Autodesk Inventor part; units mm, degrees
ref_plane "YZ Plane" through (0, 0, 0) normal (1, 0, 0) x (0, 1, 0)
ref_plane "XZ Plane" through (0, 0, 0) normal (0, 1, 0) x (-1, 0, 0)
ref_plane "XY Plane" through (0, 0, 0) normal (0, 0, 1) x (1, 0, 0)
sketch "Sketch1" plane through (0, 0, 0) normal (0, 1, 0) x (-1, 0, 0)
  line L0 (0, 0) -> (0, 10)
  line L1 (0, 10) -> (18.8, 10)
  line L2 (18.8, 10) -> (18.8, 5)
  line L3 (18.8, 5) -> (32.9, 5)
  line L4 (32.9, 5) -> (32.9, 0)
  line L5 (32.9, 0) -> (0, 0)
  dimension "d0" = 65.8
  dimension "d1" = 37.6
  dimension "d2" = 5
  dimension "d3" = 5
revolve "Revolution1" add sketch "Sketch1" angle 360 about axis through (0, 0, 0) along (0, 0, 1)
hole "Hole1" at (0, 0, 0) direction (0, 0, 1) diameter 25 end through all
chamfer "Chamfer1" distance 0.5 angle 45 4 edges at (32.9, 0, 0) (18.8, 0, 10) (32.9, 0, 5) (0, -12.5, 10)
chamfer "Chamfer2" distance 1 angle 45 1 edges at (0, -12.5, 0)
properties part number "Mesh-mounting-help" material "Nylon 6/6"
Here's how the part is built. I have some questions about the finished solid (model axes, mm). A direction names the side the tool comes from. Coordinates: 2 decimals unless noted, no trailing zeros. Order: outer loops, then holes, each group sorted by start corner. A loop starts at its lowest first (then second) coordinate and runs counter-clockwise, first axis right, second up. Notation, with made-up numbers: M 12,42 L 68,42 A10 ccw 68,52 Z; hole C 69,-18.75 d1. An arc over 180 degrees is marked long. Answer as a JSON object with one key per item and string values. Group by question number.
(1) I need wall thicknesses on probe 1 along X at (y, z) = (0, 1.25); probe 2 along Y at (x, z) = (0, 6.5). Which ranges of each line are inside material? Lowest first, please.
(2) Suppose I cut it at A-A, the plane y = 0. Please give me the cut outline in (x, z), then the cut area to 3 significant figures.
(3) Suppose I cut it at C-C, the plane z = 8.5. Please give me the cut outline in (x, y).
(4) For pin 1 (4 mm diameter, centred on x = -21, z = 5, fed in from -Y); pin 2 (5 mm diameter, centred on x = -1, y = 23, fed in from +Z); pin 3 (1.5 mm diameter, centred on x = -0.5, z = 2.5, fed in from +Y), each with a flat end and sliding along its axis, tell me the tip position at first contact or that it passes through.
(5) Which directions (+Z, -Z, +X, -X, +Y, -Y) give clear straight access to the entire face, cutting with the end or side of a thin tool? Please do faces 4 (the face through (4.08, -18.35, 7.22)), 5 (the face through (0, 14, 0)).
(6) If we mould it in two halves opening along Y, with no side actions, what happens to faces 1 (the face through (-3.755, 11.923, 5.31)), 2 (the face through (12.5, -4.3, 10)), 3 (the face through (7.13, -32.12, 2.47))? For each: released by +Y, released by -Y, zero draft, split by the parting line, or undercut.
Values found:
{
 "1": {"probe 1": "x = -32.9 to -12.5, 12.5 to 32.9", "probe 2": "y = -18.8 to -12.5, 12.5 to 18.8"},
 "2": {"outline": "M -32.9,0.5 L -32.4,0 L -13.5,0 L -12.5,1 L -12.5,9.5 L -13,10 L -18.3,10 L -18.8,9.5 L -18.8,5 L -32.4,5 L -32.9,4.5 Z; M 12.5,1 L 13.5,0 L 32.4,0 L 32.9,0.5 L 32.9,4.5 L 32.4,5 L 18.8,5 L 18.8,9.5 L 18.3,10 L 13,10 L 12.5,9.5 Z", "area": "265 mm^2"},
 "3": {"outline": "C 0,0 d37.6; hole C 0,0 d25"},
 "4": {"pin 1": "stops at y = -26.81", "pin 2": "stops at z = 5", "pin 3": "stops at y = 32.9"},
 "5": {"face 4": "+Z", "face 5": "-Z, +X, -X, +Y, -Y"},
 "6": {"face 1": "undercut", "face 2": "zero draft", "face 3": "split by the parting line"}
}
